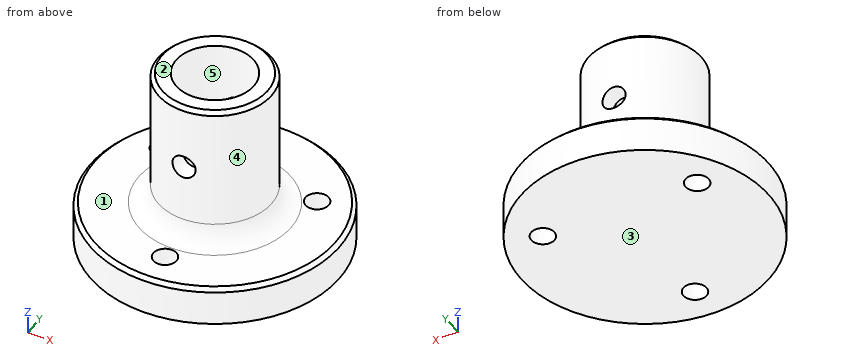
from build123d import *

# Parameters (mm, degrees)
SKETCH1_R               = 32
SKETCH1_R_2             = 3
BOSS_EXTRUDE1_DEPTH     = 10
SKETCH2_R               = 14.6
SKETCH2_R_2             = 10
BOSS_EXTRUDE2_DEPTH     = 37
CUT_EXTRUDE1_DEPTH      = 66.245689513
CUT_EXTRUDE1_DEPTH_BACK = 66.245689513
SKETCH3_R               = 3
FILLET_1_R              = 5
CHAMFER_1_SIZE          = 1


with BuildPart() as part:
    # Sketch1 → Boss-Extrude1 (new body)
    with BuildSketch(Plane.XY):
        Circle(SKETCH1_R)
        with Locations((20, 11.547005384)):
            Circle(SKETCH1_R_2, mode=Mode.SUBTRACT)
        with Locations((0, -23.094010768)):
            Circle(SKETCH1_R_2, mode=Mode.SUBTRACT)
        with Locations((-20, 11.547005384)):
            Circle(SKETCH1_R_2, mode=Mode.SUBTRACT)
    extrude(amount=BOSS_EXTRUDE1_DEPTH)

    # Sketch2 → Boss-Extrude2 (add)
    with BuildSketch(Plane.XY.offset(10)):
        Circle(SKETCH2_R)
        Circle(SKETCH2_R_2, mode=Mode.SUBTRACT)
    extrude(amount=BOSS_EXTRUDE2_DEPTH)

    # Sketch3 → Cut-Extrude1 (cut, two sides: drawn at the far end of the back side and taken through both)
    with BuildSketch(Plane(origin=(0, 0, 0), x_dir=(1, 0, 0), z_dir=(0, 1, 0)).offset(-CUT_EXTRUDE1_DEPTH_BACK)):
        with Locations(Location((0, -30, 0), (0, 0, 270))):
            Circle(SKETCH3_R)
    extrude(amount=CUT_EXTRUDE1_DEPTH + CUT_EXTRUDE1_DEPTH_BACK, mode=Mode.SUBTRACT)

    # 圆角1
    fillet_1_edges = [part.edges().sort_by_distance(p)[0] for p in [
        (-14.6, 0, 10),
    ]]
    fillet(fillet_1_edges, radius=FILLET_1_R)

    # 倒角1
    chamfer_1_edges = [part.edges().sort_by_distance(p)[0] for p in [
        (-14.6, 0, 47),
        (-32, 0, 10),
    ]]
    chamfer(chamfer_1_edges, length=CHAMFER_1_SIZE)


solid = part.part
Could you check a few things on this model? Use its own coordinates, in mm. Face numbers are marked on the shaded views. A direction names the side the tool comes from. Round coordinates to 2 decimals unless told otherwise and drop trailing zeros. Loops run counter-clockwise (first coordinate to the right, second up) from the corner with the lowest first, then second, coordinate; pieces in that order, holes last. Notation, with made-up numbers: (85, -17.75) -> (128, -17.75) arc R24 cw to (128, -7.75) -> close; hole circle Ø6 at (19.5, 21.25). An arc over 180 degrees is marked (long way). Use CSV: the item, a comma, the result in double quotes.
(1) Suppose I cut it at A-A on x = 0. Give the number of separate pieces and of enclosed holes in the cut face, plus the area to 3 significant figures.
Return value:
separate pieces,"4"
enclosed holes,"0"
area,"874 mm²"
(2) Suppose I cut it at B-B on y = 0. Write out the boundary of the cut face in (x, z), plus the area to 3 significant figures.
Return value:
outline,"(-32, 0) -> (32, 0) -> (32, 9) -> (31, 10) -> (19.6, 10) arc R5 cw to (14.6, 15) -> (14.6, 46) -> (13.6, 47) -> (10, 47) -> (10, 10) -> (-10, 10) -> (-10, 47) -> (-13.6, 47) -> (-14.6, 46) -> (-14.6, 15) arc R5 cw to (-19.6, 10) -> (-31, 10) -> (-32, 9) -> close"
area,"989 mm²"
(3) If I drill on probe 1 along Y at (x, z) = (0, 3.25); probe 2 along Z at (x, y) = (0, 13.05); probe 3 along Z at (x, y) = (-24, -6), over which ranges is the centre line in solid material (lowest first)? Write a range as [from, to].
Return value:
probe 1,"y = [-32, -26.09], [-20.09, 32]"
probe 2,"z = [0, 27], [33, 47]"
probe 3,"z = [0, 10]"
(4) Suppose I cut it at C-C on z = 30. Write out the boundary of the cut face in (x, y).
Return value:
outline,"(-3, -14.29) -> (-3, -9.54) arc R10 cw to (-3, 9.54) -> (-3, 14.29) arc R14.6 ccw to start; (3, -14.29) arc R14.6 ccw to (3, 14.29) -> (3, 9.54) arc R10 cw to (3, -9.54) -> close"
(5) Suppose I cut it at D-D on z = 11. Write out the boundary of the cut face in (x, y).
Return value:
outline,"circle Ø33.2 at (0, 0); hole circle Ø20 at (0, 0)"
(6) Will these pins go through, and if not, where does the flat tip stop? pin 1 Ø1.5 at (y, z) = (3, 10) entering from +X; pin 2 Ø1 at (x, z) = (-11, 33.5) entering from -Y; pin 3 Ø7 at (x, z) = (0, 30) entering from +Y.
Return value:
pin 1,"stops at x = 31.61"
pin 2,"stops at y = -10.14"
pin 3,"stops at y = 14.6"
(7) If we mould it in two halves opening along Y, with no side actions, what happens to the marked faces 3, 4 and 5? For each: +Y half, -Y half, draft (parallel to the pull), parting line (faces both ways), or undercut.
Return value:
face 3,"draft"
face 4,"parting line"
face 5,"undercut"
(8) For the marked faces 1 and 2, which set-ups out of +Z, -Z, +X, -X, +Y, -Y let a thin tool reach every point of the face, with its end or its side?
Return value:
face 1,"+Z"
face 2,"+Z, +X, -X, +Y, -Y"
